Part model, mm, in its own coordinate system. A direction names the side the tool comes from. Coordinates: 2 decimals unless noted, no trailing zeros. Loops run counter-clockwise (first coordinate to the right, second up) from the corner with the lowest first, then second, coordinate; pieces in that order, holes last. Notation, with made-up numbers: (75, -7.5) - (112, -7.5) arc R13 ccw to (112, 12.5) - close; hole circle Ø9 at (63.5, -12). An arc over 180 degrees is marked (long way). Use a Markdown table: item, result. Add a question column.
1) Band-saw the part on A-A (y = -9.5). Give the cut face in (x, z), plus the area to 3 significant figures.
2) Drop flat-ended pins along their axis: P1, Ø1.8, axis at x = 67.5, z = 2, coming from the +Y side; P2, Ø3, axis at y = 5.5, z = 4.5, coming from the -X side. Give the stop position or say it passes through.
3) Tool access for faces 4 (the face through (92.738, -13.177, 2.958)), 5 (the face through (96.537, -9.591, 3.042)), 6 (the face through (117, 9, 3)): list every direction of +Z, -Z, +X, -X, +Y, -Y with a clear straight run to the whole face (end or side of a thin tool).
4) Probe probe 1 along X at (y, z) = (15.5, 5.5); probe 2 along X at (y, z) = (23, 5.5); probe 3 along Y at (x, z) = (78, 3.2). List the from-to ranges inside material, lowest first. Write a range as [from, to].
5) Band-saw the part on B-B (x = 78). Give the cut face in (y, z), plus the area to 3 significant figures.
6) Pull direction X, two halves, no side cores. Call faces 1 (the face through (116.02, 18, 3)), 2 (the face through (164.5, 23, 3)), 3 (the face through (156, 26, 3)): +X half, -X half, draft (parallel to the pull), parting line (faces both ways), or undercut.
7) Band-saw the part on C-C (x = 125). Give the cut face in (y, z).
from build123d import *

# Parameters (mm, degrees)
BOSS_EXTRUDE1_DEPTH = 6
CHAMFER2_SIZE       = 0.5
CUT_EXTRUDE1_DEPTH  = 7


with BuildPart() as part:
    # Sketch1 → Boss-Extrude1 (new body)
    with BuildSketch(Plane.XY):
        with BuildLine():
            Line((116.02, 20), (116.02, 15))
            Line((116.02, 15), (114.05, 15))
            Line((114.05, 15), (114.05, 14.5))
            Line((114.05, 14.5), (114.8, 14.5))
            Line((114.8, 14.5), (114.8, 12))
            Line((114.8, 12), (116.02, 12))
            Line((116.02, 12), (116.02, 9))
            Line((116.02, 9), (118.98, 9))
            Line((118.98, 9), (118.98, 12))
            Line((118.98, 12), (120.2, 12))
            Line((120.2, 12), (120.2, 14.5))
            Line((120.2, 14.5), (120.95, 14.5))
            Line((120.95, 14.5), (120.95, 15))
            Line((120.95, 15), (118.98, 15))
            Line((118.98, 15), (118.98, 20))
            Line((118.98, 20), (148.5, 20))
            Line((148.5, 20), (148.5, 26))
            Line((148.5, 26), (164.5, 26))
            Line((164.5, 26), (164.5, 20))
            Line((164.5, 20), (166.5, 20))
            Line((166.5, 20), (166.5, 6.863840125))
            Line((166.5, 6.863840125), (88.166127224, -14.419164582))
            ThreePointArc((88.166127224, -14.419164582), (75.2601036, -1.915582926), (70.455783207, -19.230995297))
            Line((70.455783207, -19.230995297), (63.870699409, -21.020136629))
            ThreePointArc((63.870699409, -21.020136629), (37.847031663, -5.428892585), (8, 0))
            ThreePointArc((8, 0), (5.656854017, 5.656854482), (-6.59e-07, 8))
            Line((-6.59e-07, 8), (-16.5, 8))
            Line((-16.5, 8), (-16.5, 26))
            Line((-16.5, 26), (-10.5, 26))
            Line((-10.5, 26), (-10.5, 20))
            Line((-10.5, 20), (16.02, 20))
            Line((16.02, 20), (16.02, 15))
            Line((16.02, 15), (14.05, 15))
            Line((14.05, 15), (14.05, 14.5))
            Line((14.05, 14.5), (14.8, 14.5))
            Line((14.8, 14.5), (14.8, 12))
            Line((14.8, 12), (16.02, 12))
            Line((16.02, 12), (16.02, 9))
            Line((16.02, 9), (18.98, 9))
            Line((18.98, 9), (18.98, 12))
            Line((18.98, 12), (20.2, 12))
            Line((20.2, 12), (20.2, 14.5))
            Line((20.2, 14.5), (20.95, 14.5))
            Line((20.95, 14.5), (20.95, 15))
            Line((20.95, 15), (18.98, 15))
            Line((18.98, 15), (18.98, 20))
            Line((18.98, 20), (116.02, 20))
        make_face()
    extrude(amount=BOSS_EXTRUDE1_DEPTH)

    # Chamfer2
    chamfer2_edges = [part.edges().sort_by_distance(p)[0] for p in [
        (148.5, 26, 3),
        (164.5, 26, 3),
    ]]
    chamfer(chamfer2_edges, length=CHAMFER2_SIZE)

    # Sketch2 → Cut-Extrude1 (cut, through all)
    with BuildSketch(Plane.XY.offset(6)):
        Polygon((100.039498636, -11.193216334), (97.183051312, -11.969301821), (95.872096096, -7.144221882), (93.9710146, -7.660738237), (93.839919078, -7.178230243), (94.563681069, -6.981586961), (93.908203462, -4.569046991), (95.085522967, -4.249173918), (94.298949838, -1.354125954), (97.155397162, -0.578040467), (97.941970291, -3.473088431), (99.119289796, -3.153215358), (99.774767404, -5.565755328), (100.498529395, -5.369112046), (100.629624916, -5.851620039), (98.72854342, -6.368136394), align=None)
    extrude(amount=-CUT_EXTRUDE1_DEPTH, mode=Mode.SUBTRACT)


solid = part.part
Answer block:
| question | item | result |
|---|---|---|
| 1 | outline | (46.99, 0) - (67.85, 0) - (67.85, 6) - (46.99, 6) - close; (88.15, 0) - (96.51, 0) - (96.51, 6) - (88.15, 6) - close; (99.58, 0) - (106.27, 0) - (106.27, 6) - (99.58, 6) - close |
| 1 | area | 216 mm2 |
| 2 | P1 | y = 20 |
| 2 | P2 | x = 3.87 |
| 3 | face 4 | +Z, -Z, +X, -Y |
| 3 | face 5 | +Z, -Z |
| 3 | face 6 | +Z, -Z, +Y |
| 4 | probe 1 | [-16.5, 16.02], [18.98, 116.02], [118.98, 166.5] |
| 4 | probe 2 | [-16.5, -10.5], [148.5, 164.5] |
| 4 | probe 3 | [-1.55, 20] |
| 5 | outline | (-1.55, 0) - (20, 0) - (20, 6) - (-1.55, 6) - close |
| 5 | area | 129 mm2 |
| 6 | face 1 | undercut |
| 6 | face 2 | +X half |
| 6 | face 3 | draft |
| 7 | outline | (-4.41, 0) - (20, 0) - (20, 6) - (-4.41, 6) - close |
